Part model, mm, in its own coordinate system. Face numbers are marked on the shaded views. A direction names the side the tool comes from. Coordinates: 2 decimals unless noted, no trailing zeros. Loops run counter-clockwise (first coordinate to the right, second up) from the corner with the lowest first, then second, coordinate; pieces in that order, holes last. Notation, with made-up numbers: (80.5, -29) - (103.5, -29) arc R17 cw to (103.5, -15) - close; hole circle Ø5 at (34, 18.5). An arc over 180 degrees is marked (long way). Use a Markdown table: item, result. Add a question column.
1. Pull direction Z, two halves, no side cores. Call the marked faces 1, 2 and 3: pulls with the +Z half, pulls with the -Z half, needs draft (parallel to the pull), parting line crosses it, or undercut.
2. Band-saw the part on C-C, the plane y = 6.25. Give the cut face in (x, z) (3 decimals), plus the area to 3 significant figures.
3. Band-saw the part on B-B, the plane z = 5. Give the cut face in (x, y) (3 decimals), plus the area to 4 significant figures.
4. Drop flat-ended pins along their axis: pin 1 (1 mm diameter, centred on x = 20.5, z = 5.5, fed in from -Y); pin 2 (2 mm diameter, centred on x = 16, z = 5, fed in from +Y). Give the stop position or say it passes through.
5. Band-saw the part on D-D, the plane y = 1. Give the cut face in (x, z).
6. 3-axis set-ups, long thin cutter, end or side, ignore diameter. For the marked faces 4 and 5: which of +Z, -Z, +X, -X, +Y, -Y reach the whole face in a straight line?
7. Wall check: probe 1 along X at (y, z) = (6.25, 5.5); probe 2 along Z at (x, y) = (30, 6.7); probe 3 along Y at (x, z) = (27, 6). Give the ranges that are in metal, low to high. Write a range as [from, to].
8. Band-saw the part on A-A, the plane x = 10. Give the cut face in (y, z).
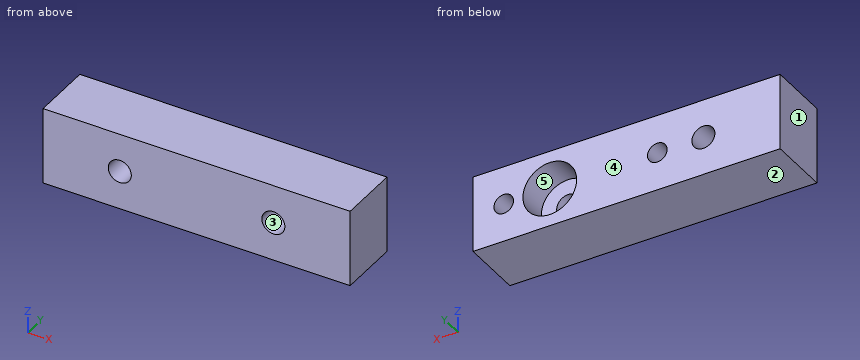
Autodesk Fusion 360 part; units mm, degrees
sketch "Skizze1" plane through (0, 0, 0) normal (0, 1, 0) x (1, 0, 0)
  line L0 (0, 0) -> (40, 0)
  line L1 (40, 0) -> (40, -5)
  line L2 (40, -5) -> (40, -10)
  line L3 (40, -10) -> (0, -10)
  line L4 (0, -10) -> (0, 0)
extrude "Extrusion1" add sketch "Skizze1" along normal blind 8
sketch "Skizze2" plane through (0, 8, 0) normal (0, 1, 0) x (-1, 0, 0)
  line L0 (0, 10) -> (-40, 10)
  line L1 (-40, 10) -> (-40, 0)
  line L2 (-40, 0) -> (0, 0)
  line L3 (0, 0) -> (0, 10)
  circle A0 centre (-10, 5) radius 1.5
  line L4 (-40, 0) -> (-40, 5)
  circle A1 centre (-36, 5) radius 1.275
  circle A2 centre (-16, 5) radius 1.275
  line L5 (-10, 5) -> (-30, 5)
  circle A3 centre (-30, 5) radius 1.5
  circle A4 centre (-30, 5) radius 3.5
  dimension "d3" = 3
  dimension "d4" = 2.55
  dimension "d5" = 2.55
  dimension "d6" = 3
  dimension "d7" = 7
extrude "Extrusion2" cut sketch "Skizze2" against normal blind 20 contours A0 | A3
extrude "Extrusion3" cut sketch "Skizze2" against normal blind 5 contours A2 L5 | A2 L5
extrude "Extrusion4" cut sketch "Skizze2" against normal blind 5 contours A1
extrude "Extrusion5" cut sketch "Skizze2" against normal blind 4 contours A4
Geometry check:
| question | item | result |
|---|---|---|
| 1 | face 1 | needs draft |
| 1 | face 2 | pulls with the -Z half |
| 1 | face 3 | undercut |
| 2 | outline | (0, 0) - (40, 0) - (40, 10) - (0, 10) - close; hole circle Ø3 at (10, 5); hole circle Ø2.55 at (16, 5); hole circle Ø7 at (30, 5); hole circle Ø2.55 at (36, 5) |
| 2 | area | 344 mm^2 |
| 3 | outline | (0, 0) - (8.5, 0) - (8.5, 8) - (0, 8) - close; (11.5, 0) - (28.5, 0) - (28.5, 4) - (26.5, 4) - (26.5, 8) - (17.275, 8) - (17.275, 3) - (14.725, 3) - (14.725, 8) - (11.5, 8) - close; (31.5, 0) - (40, 0) - (40, 8) - (37.275, 8) - (37.275, 3) - (34.725, 3) - (34.725, 8) - (33.5, 8) - (33.5, 4) - (31.5, 4) - close |
| 3 | area | 230.5 mm^2 |
| 4 | pin 1 | stops at y = 0 |
| 4 | pin 2 | stops at y = 3 |
| 5 | outline | (0, 0) - (40, 0) - (40, 10) - (0, 10) - close; hole circle Ø3 at (10, 5); hole circle Ø3 at (30, 5) |
| 6 | face 4 | +Z, -Z, +X, -X, +Y |
| 6 | face 5 | +Y |
| 7 | probe 1 | x = [0, 8.59], [11.41, 14.83], [17.17, 26.54], [33.46, 34.83], [37.17, 40] |
| 7 | probe 2 | z = [0, 1.5], [8.5, 10] |
| 7 | probe 3 | y = [0, 4] |
| 8 | outline | (0, 0) - (8, 0) - (8, 3.5) - (0, 3.5) - close; (0, 6.5) - (8, 6.5) - (8, 10) - (0, 10) - close |
